```python
from build123d import *

# Parameters (mm, degrees)
FILLET1_R = 0.75
FILLET2_R = 0.1


with BuildPart() as part:
    # Sketch1 → Revolve1 (revolve)
    with BuildSketch(Plane.XY, mode=Mode.PRIVATE) as revolve1_sk:
        Polygon((1.5, 14.15), (2.5, 14.15), (3.5, 13.15), (3.5, 12.65), (2.75, 12.15), (2.75, 10.65), (3.5, 10.15), (3.5, 7.15), (4.955, 7.15), (4.955, 1.5), (7.9, 1.5), (7.9, 0), (5.85, 0), (5.85, -4.5), (1.4, -4.5), (1.4, -9.1), (2.4, -9.1), (2.4, -10.8), (0.15, -16.9), (0.15, 0), (1.5, 0), align=None)
    revolve(revolve1_sk.sketch.rotate(Axis((0, 0, 0), (0, 1, 0)), 90), axis=Axis((0, 0, 0), (0, 1, 0)))

    # Fillet1
    fillet1_edges = [part.edges().sort_by_distance(p)[0] for p in [
        (0, -4.5, 5.85),
    ]]
    fillet(fillet1_edges, radius=FILLET1_R)

    # Fillet2
    fillet2_edges = [part.edges().sort_by_distance(p)[0] for p in [
        (0, 7.15, 4.955),
        (0, 10.15, 3.5),
    ]]
    fillet(fillet2_edges, radius=FILLET2_R)


solid = part.part
```
Geometry check sheet. Reference: the model listing, model coordinates, mm. A direction names the side the tool comes from. Give positions to 0.01 mm unless a question says otherwise; leave off trailing zeros. Order: outer loops, then holes, each group sorted by start corner. A loop starts at its lowest first (then second) coordinate and runs counter-clockwise, first axis right, second up.
1. Access from +Z, -Z, +X, -X, +Y, -Y to the whole of each face (thin tool, end or side, straight path). Record for faces 1 (the face through (3.105, 12.896, -1.615)), 2 (the face through (1.1, -4.5, -1.1)), 3 (the face through (-2.024, -9.962, -1.29)), 4 (the face through (2, 14.15, 0)), 5 (the face through (-5.34, 0.74, 5.82)).
2. Section check B-B, the plane y = 9.5. Enter the section's corners in (x, z), and give its area (3 significant figures).
3. Release check for a two-part mould opening along Y. For faces 6 (the face through (-1.488, 4.236, -4.726)), 7 (the face through (0, 0, 6)), 8 (the face through (2, -9.1, 0)) record: pulls with the +Y half, pulls with the -Y half, needs draft (parallel to the pull), parting line crosses it, or undercut.
4. Section check A-A, the plane y = -7.5. Enter the section's corners in (x, z), and give its area (3 significant figures).
5. Thickness scan on L1, parallel to X at y = 9, z = 0; L2, parallel to Y at x = -5.5, z = 4.75; L3, parallel to X at y = 10.5, z = 0 (3 decimals). Record the ranges inside material, lowest first.
6. Gauge pin test, flat ends, axial feed: pin 1 Ø6 at (y, z) = (-11.5, -1) entering from -X; pin 2 Ø8 at (x, z) = (5, 4.5) entering from -Y; pin 3 Ø5 at (x, y) = (5, -9) entering from -Z (3 decimals); pin 4 Ø2.5 at (x, z) = (0, 0) entering from +Y. Record the tip position at first contact, or that the pin passes through.
Values follow:
1. face 1: +Y
1. face 2: none
1. face 3: -Y
1. face 4: +Z, -Z, +X, -X, +Y
1. face 5: +Y, -Y
2. outline: circle Ø7 at (0, 0); hole circle Ø3 at (0, 0)
2. area: 31.4 mm2
3. face 6: needs draft
3. face 7: pulls with the -Y half
3. face 8: undercut
4. outline: circle Ø2.8 at (0, 0); hole circle Ø0.3 at (0, 0)
4. area: 6.09 mm2
5. L1: x = -3.5 to -1.5, 1.5 to 3.5
5. L2: y = 0 to 1.5
5. L3: x = -2.975 to -1.5, 1.5 to 2.975
6. pin 1: stops at x = -2.4
6. pin 2: stops at y = -4.5
6. pin 3: passes through
6. pin 4: stops at y = 0
